CAD build for the part. Positions are in the model's coordinates, mm. Coordinates: 2 decimals unless noted, no trailing zeros. Write each loop counter-clockwise with the first axis right and the second up, starting at its lowest first coordinate (ties: lowest second). Pieces come first, ordered by that corner, then holes. Notation, with made-up numbers: M -24.5,56.5 L 21.5,56.5 A16 cw 21.5,70.5 Z; hole C -24,2 d2. An arc over 180 degrees is marked long. Put each result on its own line as item: value. Start each with the question number.
Autodesk Inventor part; units mm, degrees
ref_plane "YZ Plane" through (0, 0, 0) normal (1, 0, 0) x (0, 1, 0)
ref_plane "XZ Plane" through (0, 0, 0) normal (0, 1, 0) x (-1, 0, 0)
ref_plane "XY Plane" through (0, 0, 0) normal (0, 0, 1) x (1, 0, 0)
sketch "Sketch1" plane through (0, 0, 0) normal (0, 0, 1) x (1, 0, 0)
  line L0 (27.5, 166.3577) -> (122.5, 166.3577)
  line L1 (122.5, 166.3577) -> (122.5, 121.3577)
  line L2 (122.5, 121.3577) -> (27.5, 121.3577)
  line L3 (27.5, 121.3577) -> (27.5, 166.3577)
  line L4 (52.5, 100.1) -> (97.5, 100.1)
  line L5 (97.5, 100.1) -> (97.5, 45.1)
  line L6 (97.5, 45.1) -> (52.5, 45.1)
  line L7 (52.5, 45.1) -> (52.5, 100.1)
  line L8 (0, 0) -> (150, 0)
  line L9 (0, 200) -> (150, 200)
  line L10 (0, 153.4) -> (0, 120)
  line L11 (0, 80) -> (0, 0)
  line L12 (0, 153.4) -> (0, 200)
  line L13 (0, 120) -> (-30, 120)
  line L14 (-30, 120) -> (-30, 80)
  line L15 (-30, 80) -> (0, 80)
  line L16 (-20, 110) -> (-10, 110)
  line L17 (-10, 110) -> (-10, 90)
  line L18 (-10, 90) -> (-20, 90)
  line L19 (-20, 90) -> (-20, 110)
  line L20 (150, 200) -> (150, 0)
  dimension "d0" = 150
  dimension "d49" = 200
  dimension "d50" = 40
  dimension "d51" = 80
  dimension "d52" = 10
  dimension "d53" = 95
  dimension "d54" = 45
  dimension "d55" = 45
  dimension "d56" = 55
extrude "Extrusion1" add sketch "Sketch1" along normal blind 3 contours L11 L15 L14 L13 L10 L12 L9 L20 L8 | L16 L17 L18 L19
sketch "Sketch2" plane through (0, 0, 3) normal (0, 0, 1) x (1, 0, 0)
  line L0 (-30, 80.2736) -> (0, 80.2736)
  line L1 (-20, 110.2736) -> (-10, 110.2736)
  line L2 (-10, 110.2736) -> (-10, 90.2736)
  line L3 (-10, 90.2736) -> (-20, 90.2736)
  line L4 (-20, 90.2736) -> (-20, 110.2736)
  line L5 (0, 117.7458) -> (0, 120.2736)
  point P0 (0, 0)
extrude "Extrusion2" cut sketch "Sketch2" against normal blind 3
properties part number "depan"
(1) Drop flat-ended pins along their axis: pin 1 (1.5 mm diameter, centred on x = -22, z = 1.5, fed in from +Y); pin 2 (1.5 mm diameter, centred on x = 83.5, z = 0.5, fed in from -Y); pin 3 (1 mm diameter, centred on x = -2, y = 32, fed in from -Z). Give the stop position or say it passes through.
(2) Slice it at B-B, the plane x = 103. Write the cut outline in (y, z), then the cut area to 3 significant figures.
(3) Slice it at D-D, the plane y = 53.5. Write the cut outline in (x, z), then the cut area to 3 significant figures.
(4) Drill centre lines: line 1 (Y direction, x = 74, z = 2.85); line 2 (X direction, y = 155.5, z = 1.3); line 3 (Y direction, x = 38, z = 2.75). Where is each one in solid material? Low to high. Write a range as [from, to].
(5) Slice it at A-A, the plane y = 95. Write the cut outline in (x, z), then the cut area to 3 significant figures.
(6) Slice it at C-C, the plane z = 1.9. Write the cut outline in (x, y).
Result set:
1. pin 1: stops at y = 120
1. pin 2: stops at y = 0
1. pin 3: passes through
2. outline: M 0,0 L 121.36,0 L 121.36,3 L 0,3 Z; M 166.36,0 L 200,0 L 200,3 L 166.36,3 Z
2. area: 465 mm^2
3. outline: M 0,0 L 52.5,0 L 52.5,3 L 0,3 Z; M 97.5,0 L 150,0 L 150,3 L 97.5,3 Z
3. area: 315 mm^2
4. line 1: y = [0, 45.1], [100.1, 121.36], [166.36, 200]
4. line 2: x = [0, 27.5], [122.5, 150]
4. line 3: y = [0, 121.36], [166.36, 200]
5. outline: M -30,0 L -20,0 L -20,3 L -30,3 Z; M -10,0 L 52.5,0 L 52.5,3 L -10,3 Z; M 97.5,0 L 150,0 L 150,3 L 97.5,3 Z
5. area: 375 mm^2
6. outline: M -30,80 L 0,80 L 0,0 L 150,0 L 150,200 L 0,200 L 0,120 L -30,120 Z; hole M -20,90.27 L -10,90.27 L -10,110.27 L -20,110.27 Z; hole M 27.5,121.36 L 122.5,121.36 L 122.5,166.36 L 27.5,166.36 Z; hole M 52.5,45.1 L 97.5,45.1 L 97.5,100.1 L 52.5,100.1 Z
